from build123d import *

# Parameters (mm, degrees)
SKETCH1_W = 10
SKETCH1_H = 478


with BuildPart() as part:
    # Sketch1 → Revolve1 (revolve)
    with BuildSketch(Plane.XY, mode=Mode.PRIVATE) as revolve1_sk:
        with Locations((-5, 0)):
            Rectangle(SKETCH1_W, SKETCH1_H)
    revolve(revolve1_sk.sketch.rotate(Axis((0, -239, 0), (0, 1, 0)), 180), axis=Axis((0, -239, 0), (0, 1, 0)))

    # Sketch2 → Revolve2 (revolve)
    with BuildSketch(Plane.XY):
        with BuildLine():
            Line((-10, 239), (0, 239))
            Line((0, 239), (0, 265.180339887))
            ThreePointArc((0, 265.180339887), (-14.012585384, 255.532671234), (-10, 239))
        make_face()
    revolve2 = revolve(axis=Axis((0, 0, 0), (0, 1, 0)))

    # Mirror1: Revolve2 across plane
    add(revolve2.mirror(Plane.ZX))


solid = part.part
Verification items for the finished model (mm, model axes). Coordinates: 2 decimals unless noted, no trailing zeros. Order: outer loops, then holes, each group sorted by start corner. A loop starts at its lowest first (then second) coordinate and runs counter-clockwise, first axis right, second up. Notation, with made-up numbers: M 41,4.25 L 67,4.25 A25 cw 67,37.25 Z; hole C -16,-37 d2. An arc over 180 degrees is marked long. One line per item, written item: value. Start each with the question number.
Item 1: Scan lines: probe 1 along X at (y, z) = (-115.5, -1); probe 2 along Y at (x, z) = (-5.75, -12.25); probe 3 along Y at (x, z) = (12, -4.25). Record each from-to range of solid material in increasing order.
Item 2: Gauge pin test, flat ends, axial feed: pin 1 (8 mm diameter, centred on y = -25, z = 7, fed in from +X); pin 2 (2 mm diameter, centred on y = 166.5, z = 1, fed in from -X); pin 3 (6 mm diameter, centred on y = -33.5, z = 2.5, fed in from +X). Record the tip position at first contact, or that the pin passes through.
Item 3: Sectioned sample at C-C (y = 21.5). Enter the section's corners in (x, z).
Item 4: Sectioned sample at B-B (z = 0). Enter the section's corners in (x, y), then the cut area to 3 significant figures.
Item 5: Sectioned sample at A-A (x = 0). Enter the section's corners in (y, z).
Conclusion:
1. probe 1: x = -9.95 to 9.95
1. probe 2: y = -256.65 to -243.71, 243.71 to 256.65
1. probe 3: y = -258.11 to -242.25, 242.25 to 258.11
2. pin 1: stops at x = 9.54
2. pin 2: stops at x = -10
2. pin 3: stops at x = 10
3. outline: C 0,0 d20
4. outline: M -10,-239 A15 ccw long 10,-239 L 10,239 A15 ccw long -10,239 Z
4. area: 10,900 mm^2
5. outline: M -239,-10 L 239,-10 A15 ccw long 239,10 L -239,10 A15 ccw long Z
